Read the model definition and answer for the solid it produces. Units are mm, in the model's axes. Give positions to 0.01 mm unless a question says otherwise; leave off trailing zeros. Order: outer loops, then holes, each group sorted by start corner. A loop starts at its lowest first (then second) coordinate and runs counter-clockwise, first axis right, second up. Notation, with made-up numbers: (-16.5, -27) -> (7.5, -27) arc R20 ccw to (7.5, 7) -> close; hole circle Ø5 at (-32, 50.5). An arc over 180 degrees is marked (long way). One line per item, written item: value. Start each with the question number.
from build123d import *

# Parameters (mm, degrees)
F1_W     = 116
F1_H     = 90
F2_DEPTH = 1
F4_W     = 116
F4_H     = 58.6666666667
F5_DEPTH = 3
F3_W     = 8
F3_H     = 88
F3_W_2   = 6
F3_W_3   = 3
F3_W_4   = 11
F3_W_5   = 24
F6_DEPTH = 1


with BuildPart() as f2:
    # F1 (on Top) → F2 (new body)
    with BuildSketch(Plane.XY):
        Rectangle(F1_W, F1_H)
    extrude(amount=F2_DEPTH)

    # F4 (on face) → F5 (cut)
    with BuildSketch(Plane.XY.offset(1)):
        Rectangle(F4_W, F4_H)
    extrude(amount=F5_DEPTH, mode=Mode.SUBTRACT)

    # F3 (on face) → F6 (cut)
    with BuildSketch(Plane.XY.offset(1)):
        with Locations((-53, 0)):
            Rectangle(F3_W, F3_H)
        with Locations((-45, 0)):
            Rectangle(F3_W_2, F3_H)
        with Locations((-38, 0)):
            Rectangle(F3_W_2, F3_H)
        with Locations((-31, 0)):
            Rectangle(F3_W_2, F3_H)
        with Locations((-24, 0)):
            Rectangle(F3_W_2, F3_H)
        with Locations((-17, 0)):
            Rectangle(F3_W_2, F3_H)
        with Locations((-10, 0)):
            Rectangle(F3_W_2, F3_H)
        with Locations((-3, 0)):
            Rectangle(F3_W_2, F3_H)
        with Locations((2.5, 0)):
            Rectangle(F3_W_3, F3_H)
        with Locations((6.5, 0)):
            Rectangle(F3_W_3, F3_H)
        with Locations((14.5, 0)):
            Rectangle(F3_W_4, F3_H)
        with Locations((26.5, 0)):
            Rectangle(F3_W_4, F3_H)
        with Locations((45, 0)):
            Rectangle(F3_W_5, F3_H)
    extrude(amount=-F6_DEPTH, mode=Mode.SUBTRACT)


solid = f2.part
Item 1: Find section B-B on z = 0.85. Count the separate pieces of the cut face and the enclosed holes in it, then the cut area to 3 significant figures.
Item 2: Find the intervals of material crossed by line 1 (Y direction, x = -51, z = 0.35), in increasing order. Write a range as from..to.
Item 3: Find section A-A on x = -11. Write down the section's boundary in (y, z).
Checks:
1. separate pieces: 1
1. enclosed holes: 13
1. area: 1,460 mm2
2. line 1: -45..-44, 44..45
3. outline: (-45, 0) -> (-44, 0) -> (-44, 1) -> (-45, 1) -> close; (44, 0) -> (45, 0) -> (45, 1) -> (44, 1) -> close
